from build123d import *

# Parameters (mm, degrees)
OUTSIDE_EXTRUDE_DEPTH = 3.3
CUT_EXTRUDE4_DEPTH    = 1.7


with BuildPart() as part:
    # Sketch1 → Outside-extrude (new body)
    with BuildSketch(Plane(origin=(0, 0, 0), x_dir=(1, 0, 0), z_dir=(0, 1, 0))):
        with BuildLine():
            Line((-82.65, 64.5), (82.65, 64.5))
            ThreePointArc((82.65, 64.5), (87.140128061, 62.640128061), (89, 58.15))
            Line((89, 58.15), (89, -58.15))
            ThreePointArc((89, -58.15), (87.140128061, -62.640128061), (82.65, -64.5))
            Line((82.65, -64.5), (-82.65, -64.5))
            ThreePointArc((-82.65, -64.5), (-87.140128061, -62.640128061), (-89, -58.15))
            Line((-89, -58.15), (-89, 58.15))
            ThreePointArc((-89, 58.15), (-87.140128061, 62.640128061), (-82.65, 64.5))
        make_face()
        with BuildLine():
            Line((-79.5, 49.25), (79.5, 49.25))
            ThreePointArc((79.5, 49.25), (80.914213562, 48.664213562), (81.5, 47.25))
            Line((81.5, 47.25), (81.5, -47.25))
            ThreePointArc((81.5, -47.25), (80.914213562, -48.664213562), (79.5, -49.25))
            Line((79.5, -49.25), (-79.5, -49.25))
            ThreePointArc((-79.5, -49.25), (-80.914213562, -48.664213562), (-81.5, -47.25))
            Line((-81.5, -47.25), (-81.5, 47.25))
            ThreePointArc((-81.5, 47.25), (-80.914213562, 48.664213562), (-79.5, 49.25))
        make_face(mode=Mode.SUBTRACT)
    extrude(amount=OUTSIDE_EXTRUDE_DEPTH)

    # Sketch2 → Cut-Extrude4 (cut)
    with BuildSketch(Plane(origin=(0, 0, 0), x_dir=(1, 0, 0), z_dir=(0, 1, 0))):
        Polygon((-15.5, -58.5), (-15.5, -60.5), (15.5, -60.5), (15.5, -58.75), (85.5, -58.75), (85.5, 53.5), (-85.5, 53.5), (-85.5, -58.5), align=None)
    extrude(amount=CUT_EXTRUDE4_DEPTH, mode=Mode.SUBTRACT)


solid = part.part
Geometry: final body of the model. Coordinates: model frame, mm. Give positions to 0.01 mm unless a question says otherwise; leave off trailing zeros. Write each loop counter-clockwise with the first axis right and the second up, starting at its lowest first coordinate (ties: lowest second). Pieces come first, ordered by that corner, then holes. Notation, with made-up numbers: (67, -5) - (90, -5) arc R16 cw to (90, 22) - close; hole circle Ø3 at (22, -17.75). An arc over 180 degrees is marked (long way). Return JSON: item names as keys, results as strings. Group by question number.
1) Mould query, pull axis Z, two halves, no side actions, for faces 1 (the flat face through (0, 1.7, 50)), 2 (the flat face through (-89, 2, 1)), 3 (the cylindrical face through (-87.19, 1.63, -62.59)). Classes: released by +Z, released by -Z, zero draft, split by the parting line, or undercut.
2) First-contact query: P1, Ø0.8, axis at y = 1, z = 59.5, coming from the +X side; P2, Ø1.4, axis at y = 1, z = 59.5, coming from the -X side. Flat tips, straight axial feed; report the tip coordinate or a pass-through.
3) Section B-B on z = 40.5. Return the cut outline in (x, y), plus the area to 3 significant figures.
4) Line query: line 1 (X direction, y = 0.95, z = 1); line 2 (Z direction, x = 45.5, y = 2.4); line 3 (Z direction, x = -50.5, y = 1.2). Output: solid intervals per line, ascending.
5) Section D-D on z = 55. Return the cut outline in (x, y), plus the area to 3 significant figures.
6) Section A-A on x = -76. Return the cut outline in (y, z).
7) Section C-C on y = 1. Return the cut outline in (x, z), plus the area to 3 significant figures.
Filled in:
{
 "1": {"face 1": "undercut", "face 2": "zero draft", "face 3": "released by -Z"},
 "2": {"P1": "stops at x = 88.93", "P2": "stops at x = -88.97"},
 "3": {"outline": "(-89, 0) - (-85.5, 0) - (-85.5, 1.7) - (-81.5, 1.7) - (-81.5, 3.3) - (-89, 3.3) - close; (81.5, 1.7) - (85.5, 1.7) - (85.5, 0) - (89, 0) - (89, 3.3) - (81.5, 3.3) - close", "area": "35.9 mm^2"},
 "4": {"line 1": "x = -89 to -85.5, 85.5 to 89", "line 2": "z = -64.5 to -49.25, 49.25 to 64.5", "line 3": "z = -64.5 to -53.5, 58.5 to 64.5"},
 "5": {"outline": "(-89, 0) - (-85.5, 0) - (-85.5, 1.7) - (85.5, 1.7) - (85.5, 0) - (89, 0) - (89, 3.3) - (-89, 3.3) - close", "area": "297 mm^2"},
 "6": {"outline": "(0, -64.5) - (3.3, -64.5) - (3.3, -49.25) - (1.7, -49.25) - (1.7, -53.5) - (0, -53.5) - close; (0, 58.5) - (1.7, 58.5) - (1.7, 49.25) - (3.3, 49.25) - (3.3, 64.5) - (0, 64.5) - close"},
 "7": {"outline": "(-89, -58.15) arc R6.35 ccw to (-82.65, -64.5) - (82.65, -64.5) arc R6.35 ccw to (89, -58.15) - (89, 58.15) arc R6.35 ccw to (82.65, 64.5) - (-82.65, 64.5) arc R6.35 ccw to (-89, 58.15) - close; hole (-85.5, -53.5) - (85.5, -53.5) - (85.5, 58.75) - (15.5, 58.75) - (15.5, 60.5) - (-15.5, 60.5) - (-15.5, 58.5) - (-85.5, 58.5) - close", "area": "3,700 mm^2"}
}
